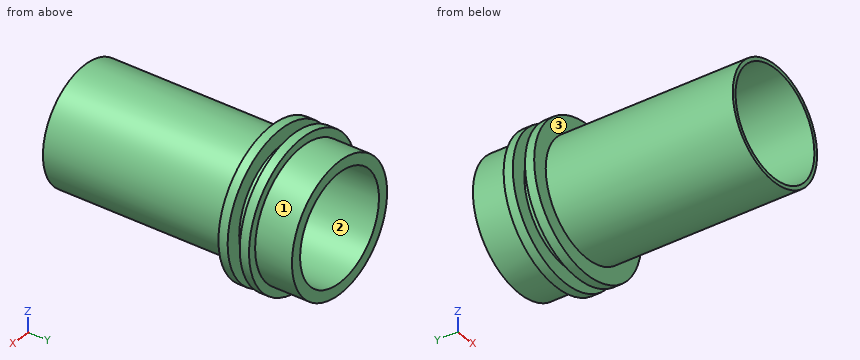
Autodesk Inventor part; units mm, degrees
ref_plane "YZ Plane" through (0, 0, 0) normal (1, 0, 0) x (0, 1, 0)
ref_plane "XZ Plane" through (0, 0, 0) normal (0, 1, 0) x (-1, 0, 0)
ref_plane "XY Plane" through (0, 0, 0) normal (0, 0, 1) x (1, 0, 0)
sketch "Sketch1" plane through (0, 0, 0) normal (0, 1, 0) x (-1, 0, 0)
  circle A0 centre (0, 0) radius 7.75
  dimension "d0" = 15.5
extrude "Extrusion1" add sketch "Sketch1" along normal blind 25.4
sketch "Sketch2" plane through (0, 25.4, 0) normal (0, 1, 0) x (1, 0, 0)
  circle A0 centre (0, 0) radius 7.75
  circle A1 centre (0, 0) radius 9.875
  dimension "d3" = 19.75
extrude "Extrusion2" add sketch "Sketch2" along normal blind 1.25 contours A0 | A1
sketch "Sketch3" plane through (0, 26.65, 0) normal (0, 1, 0) x (1, 0, 0)
  circle A0 centre (0, 0) radius 9.875
  circle A1 centre (0, 0) radius 7.75
  dimension "d6" = 15.5
extrude "Extrusion3" add sketch "Sketch3" along normal blind 1.65 contours A1
sketch "Sketch4" plane through (0, 28.3, 0) normal (0, 1, 0) x (1, 0, 0)
  circle A0 centre (0, 0) radius 7.75
  circle A1 centre (0, 0) radius 9.875
  dimension "d9" = 19.75
extrude "Extrusion4" add sketch "Sketch4" along normal blind 1.25 contours A0 | A1
sketch "Sketch5" plane through (0, 29.55, 0) normal (0, 1, 0) x (1, 0, 0)
  circle A0 centre (0, 0) radius 9.875
  circle A1 centre (0, 0) radius 8.75
  dimension "d12" = 17.5
extrude "Extrusion5" add sketch "Sketch5" along normal blind 5 contours A1
thread "Thread1"
hole "Hole1" at (0, 0, 0) direction (0, 1, 0) diameter 14.5 end through all
properties part number "Plunger" material "ABS Plastic"
Design review of the part built by this model. Coordinates are the model's own, in mm. Face numbers are marked on the shaded views. Give positions to 0.01 mm unless a question says otherwise; leave off trailing zeros. Loops run counter-clockwise (first coordinate to the right, second up) from the corner with the lowest first, then second, coordinate; pieces in that order, holes last. Notation, with made-up numbers: (-23, 76) -> (18, 76) arc R23 ccw to (18, 101) -> close; hole circle Ø9 at (-38, 29.25). An arc over 180 degrees is marked (long way). One line per item, written item: value.
Q1. For pin 1 Ø3 at (x, z) = (7.5, -1.5) entering from -Y; pin 2 Ø6 at (y, z) = (22, -5.5) entering from +X; pin 3 Ø3 at (x, y) = (0.5, 22.5) entering from +Z; pin 4 Ø6 at (y, z) = (19.5, -1.5) entering from +X, all flat-tipped, find the tip position at first contact; note any pin that passes through.
Numbers:
pin 1: stops at y = 0
pin 2: stops at x = 7.34
pin 3: stops at z = 7.75
pin 4: stops at x = 7.75
Q2. For L1, parallel to Z at x = 0, y = 19; L2, parallel to Z at x = 0.25, y = 31; L3, parallel to Y at x = -1, z = -8.75, list the stretches that pass through material, from the lowest coordinate up.
Numbers:
L1: z = -7.75 to -7.25, 7.25 to 7.75
L2: z = -8.75 to -7.25, 7.25 to 8.75
L3: y = 25.4 to 26.65, 28.3 to 29.55
Q3. We need section A-A on x = 0. Give the boundary of the cut face in (y, z) (3 decimals), and give its area (3 significant figures).
Numbers:
outline: (0, -7.75) -> (25.4, -7.75) -> (25.4, -9.875) -> (26.65, -9.875) -> (26.65, -7.75) -> (28.3, -7.75) -> (28.3, -9.875) -> (29.55, -9.875) -> (29.55, -8.75) -> (34.55, -8.75) -> (34.55, -7.25) -> (0, -7.25) -> close; (0, 7.25) -> (34.55, 7.25) -> (34.55, 8.75) -> (29.55, 8.75) -> (29.55, 9.875) -> (28.3, 9.875) -> (28.3, 7.75) -> (26.65, 7.75) -> (26.65, 9.875) -> (25.4, 9.875) -> (25.4, 7.75) -> (0, 7.75) -> close
area: 55.2 mm^2
Q4. We need section C-C on y = 29. Give the boundary of the cut face in (x, z) (3 decimals).
Numbers:
outline: circle Ø19.75 at (0, 0); hole circle Ø14.5 at (0, 0)
Q5. We need section D-D on z = -8.25. Give the boundary of the cut face in (x, y), and give its area (3 significant figures).
Numbers:
outline: (-5.43, 25.4) -> (5.43, 25.4) -> (5.43, 26.65) -> (-5.43, 26.65) -> close; (-5.43, 28.3) -> (5.43, 28.3) -> (5.43, 29.55) -> (2.92, 29.55) -> (2.92, 34.55) -> (-2.92, 34.55) -> (-2.92, 29.55) -> (-5.43, 29.55) -> close
area: 56.3 mm^2
Q6. Draft analysis for pull direction Z (two halves, no side actions). For the marked faces 1, 2 and 3, state which applies: pulls with the +Z half, pulls with the -Z half, needs draft (parallel to the pull), parting line crosses it, or undercut.
Numbers:
face 1: parting line crosses it
face 2: undercut
face 3: needs draft
Q7. We need section B-B on z = 0. Give the boundary of the cut face in (x, y) (3 decimals).
Numbers:
outline: (-9.875, 25.4) -> (-7.75, 25.4) -> (-7.75, 0) -> (-7.25, 0) -> (-7.25, 34.55) -> (-8.75, 34.55) -> (-8.75, 29.55) -> (-9.875, 29.55) -> (-9.875, 28.3) -> (-7.75, 28.3) -> (-7.75, 26.65) -> (-9.875, 26.65) -> close; (7.25, 0) -> (7.75, 0) -> (7.75, 25.4) -> (9.875, 25.4) -> (9.875, 26.65) -> (7.75, 26.65) -> (7.75, 28.3) -> (9.875, 28.3) -> (9.875, 29.55) -> (8.75, 29.55) -> (8.75, 34.55) -> (7.25, 34.55) -> close
